Autodesk Inventor part; units mm, degrees
ref_plane "YZ Plane" through (0, 0, 0) normal (1, 0, 0) x (0, 1, 0)
ref_plane "XZ Plane" through (0, 0, 0) normal (0, 1, 0) x (-1, 0, 0)
ref_plane "XY Plane" through (0, 0, 0) normal (0, 0, 1) x (1, 0, 0)
sketch "Sketch1" plane through (0, 0, 0) normal (0, 0, 1) x (1, 0, 0)
  line L0 (0, 0) -> (25.981, 0)
  line L1 (0, 16) -> (10, 16)
  line L2 (10, 16) -> (10, 18.5)
  line L3 (10, 18.5) -> (25, 18.5)
  line L4 (0, 22.5) -> (0, 16)
  line L5 (2, 22.5) -> (2, 42.5)
  line L6 (2, 42.5) -> (8, 42.5)
  line L7 (8, 42.5) -> (8, 27.5)
  line L8 (8, 27.5) -> (25, 27.5)
  line L9 (25, 27.5) -> (25, 18.5)
  line L10 (0, 22.5) -> (2, 22.5)
  dimension "d0" = 32
  dimension "d2" = 37
  dimension "d5" = 15
  dimension "d7" = 6
  dimension "d9" = 85
  dimension "d11" = 55
  dimension "d12" = 45
  dimension "d13" = 25
  dimension "d14" = 8
revolve "Revolution1" add sketch "Sketch1" angle 360 about axis through (0, 0, 0) along (1, 0, 0)
fillet "Fillet1" radius 2 3 edges at (2, -22.5, 0) (10, -18.5, 0) (8, -27.5, 0)
chamfer "Chamfer2" distance 1 angle 45 2 edges at (25, -27.5, 0) (2, -42.5, 0)
properties part number "CoverInput"
Could you check a few things on this model? Use its own coordinates, in mm. A direction names the side the tool comes from. Round coordinates to 2 decimals unless told otherwise and drop trailing zeros. Order: outer loops, then holes, each group sorted by start corner. A loop starts at its lowest first (then second) coordinate and runs counter-clockwise, first axis right, second up. Notation, with made-up numbers: M 80.25,13.5 L 109.25,13.5 A18 cw 109.25,46.5 Z; hole C 39,34.25 d1. An arc over 180 degrees is marked long. One line per question, with ' | ' between items. Start each with the question number.
(1) For P1, Ø12, axis at y = 32.5, z = -18, coming from the +X side; P2, Ø5, axis at x = 3, z = 33, coming from the +Y side; P3, Ø4, axis at x = 22.5, z = 22.5, coming from the -Y side, each with a flat end and sliding along its axis, tell me the tip position at first contact or that it passes through.
(2) Suppose I cut it at D-D on x = 22.5. List the corners of the cut face in (y, z) for me.
(3) For faces 1 (the face through (8, -29, -9)), 2 (the face through (0, -5.3, 15.3)), which set-ups out of +Z, -Z, +X, -X, +Y, -Y let a thin tool reach every point of the face, with its end or its side?
(4) Thinking about a two-plate mould opening in Y: for faces 3 (the face through (18.59, -4.01, -18.06)), 4 (the face through (2, 18, -18)), 5 (the face through (17.098, -5.961, -26.846)), which applies, +Y half, -Y half, draft (parallel to the pull), parting line (faces both ways), or undercut?
(5) Please list where these lines run through material, in increasing order: line 1 along Z through (x, y) = (22, 0); line 2 along Z through (x, y) = (3, 0); line 3 along X through (y, z) = (-30, -26.5).
(6) Suppose I cut it at C-C on x = 6.25. List the corners of the cut face in (y, z) for me.
Geometry results:
1) P1: x = 8 | P2: y = 29.6 | P3: y = -18.33
2) outline: C 0,0 d55; hole C 0,0 d37
3) face 1: +X | face 2: +Z, -Z, -X, +Y, -Y
4) face 3: undercut | face 4: draft | face 5: parting line
5) line 1: -27.5 to -18.5, 18.5 to 27.5 | line 2: -42.5 to -16, 16 to 42.5 | line 3: 2 to 8
6) outline: C 0,0 d85; hole C 0,0 d32
